Autodesk Inventor part; units mm, degrees
ref_plane "YZ Plane" through (0, 0, 0) normal (1, 0, 0) x (0, 1, 0)
ref_plane "XZ Plane" through (0, 0, 0) normal (0, 1, 0) x (-1, 0, 0)
ref_plane "XY Plane" through (0, 0, 0) normal (0, 0, 1) x (1, 0, 0)
sketch "Sketch1" plane through (0, 0, 0) normal (0, 0, 1) x (1, 0, 0)
  point P0 (0, 0)
sketch "Sketch2" plane through (0, 0, 0) normal (0, 1, 0) x (-1, 0, 0)
  line L0 (14.6, 28.7) -> (-14.6, 28.7)
  line L1 (-15.6, 27.7) -> (-15.6, -27.7)
  line L2 (-14.6, -28.7) -> (14.6, -28.7)
  line L3 (15.6, -27.7) -> (15.6, 27.7)
  line L4 (15.6, 28.7) -> (-15.6, -28.7) construction
  line L5 (-15.6, 28.7) -> (15.6, -28.7) construction
  arc A0 (15.6, 27.7) -> (14.6, 28.7) centre (14.6, 27.7) ccw
  arc A1 (-14.6, 28.7) -> (-15.6, 27.7) centre (-14.6, 27.7) ccw
  arc A2 (14.6, -28.7) -> (15.6, -27.7) centre (14.6, -27.7) ccw
  arc A3 (-15.6, -27.7) -> (-14.6, -28.7) centre (-14.6, -27.7) ccw
  circle A4 centre (12.6, 26.2) radius 1.5
  line L6 (0, 28.7) -> (0, -28.7) construction
  line L7 (15.6, 0) -> (-15.6, 0) construction
  circle A5 centre (12.6, -26.2) radius 1.5
  circle A6 centre (-12.6, 26.2) radius 1.5
  circle A7 centre (-12.6, -26.2) radius 1.5
  line L8 (1.792, 7.3985) -> (1.792, -6.1335) construction
  line L9 (1.792, -6.1335) -> (-36.4686, -6.1335) construction
  line L10 (-36.4686, -6.1335) -> (-36.4686, 7.3985) construction
  line L11 (-36.4686, 7.3985) -> (1.792, 7.3985) construction
  point P0 (0, 0)
  dimension "d0" = 31.2
  dimension "d1" = 57.4
  dimension "d2" = 1
  dimension "d3" = 3
  dimension "d4" = 3
  dimension "d5" = 2.5
extrude "Extrusion1" add sketch "Sketch2" along normal blind 1
properties part number "esp8266_footprint"
Here's how the part is built. I have some questions about the finished solid (model axes, mm). Round coordinates to 2 decimals unless told otherwise and drop trailing zeros. Loops run counter-clockwise (first coordinate to the right, second up) from the corner with the lowest first, then second, coordinate; pieces in that order, holes last. Notation, with made-up numbers: (59.5, 22.5) -> (68.5, 22.5) arc R34 ccw to (68.5, 59.5) -> close; hole circle Ø4 at (49.25, 31). An arc over 180 degrees is marked (long way). Answer as CSV lines item,"result". Start each with the question number.
1. Imagine slicing it at C-C on z = -26.2. Write out the boundary of the cut face in (x, y).
2. I'm going to push flat-ended pins straight in: P1, Ø1.8, axis at x = 12.6, z = 26.2, coming from the +Y side; P2, Ø10, axis at x = 1.5, z = -17.5, coming from the -Y side. Where does each tip first touch, or does it pass through?
3. Imagine slicing it at B-B on y = 0.8. Write out the boundary of the cut face in (x, z), plus the area to 3 significant figures.
4. If we mould it in two halves opening along X, with no side actions, what happens to faces 1 (the face through (14.1, 0.49, 26.13)), 2 (the face through (15.6, 0.5, 0.4)), 3 (the face through (0, 0, 0))? For each: pulls with the +X half, pulls with the -X half, needs draft (parallel to the pull), parting line crosses it, or undercut.
5. I need wall thicknesses on probe 1 along Z at (x, y) = (12.6, 0.55); probe 2 along X at (y, z) = (0.35, 26); probe 3 along Z at (x, y) = (-13, 0.8). Which ranges of each line are inside material? Lowest first, please. Write a range as from..to.
6. Imagine slicing it at A-A on x = 12.6. Write out the boundary of the cut face in (y, z).
Solution:
1,outline,"(-15.6, 0) -> (-14.1, 0) -> (-14.1, 1) -> (-15.6, 1) -> close; (-11.1, 0) -> (11.1, 0) -> (11.1, 1) -> (-11.1, 1) -> close; (14.1, 0) -> (15.6, 0) -> (15.6, 1) -> (14.1, 1) -> close"
2,P1,"through"
2,P2,"y = 0"
3,outline,"(-15.6, -27.7) arc R1 ccw to (-14.6, -28.7) -> (14.6, -28.7) arc R1 ccw to (15.6, -27.7) -> (15.6, 27.7) arc R1 ccw to (14.6, 28.7) -> (-14.6, 28.7) arc R1 ccw to (-15.6, 27.7) -> close; hole circle Ø3 at (-12.6, -26.2); hole circle Ø3 at (-12.6, 26.2); hole circle Ø3 at (12.6, -26.2); hole circle Ø3 at (12.6, 26.2)"
3,area,"1,760 mm²"
4,face 1,"undercut"
4,face 2,"pulls with the +X half"
4,face 3,"needs draft"
5,probe 1,"-28.7..-27.7, -24.7..24.7, 27.7..28.7"
5,probe 2,"-15.6..-14.09, -11.11..11.11, 14.09..15.6"
5,probe 3,"-28.7..-27.65, -24.75..24.75, 27.65..28.7"
6,outline,"(0, -28.7) -> (1, -28.7) -> (1, -27.7) -> (0, -27.7) -> close; (0, -24.7) -> (1, -24.7) -> (1, 24.7) -> (0, 24.7) -> close; (0, 27.7) -> (1, 27.7) -> (1, 28.7) -> (0, 28.7) -> close"
